Source: CAD feature listing. Evaluate the final solid. Frame: model axes, mm. A direction names the side the tool comes from. Round coordinates to 2 decimals unless told otherwise and drop trailing zeros. Order: outer loops, then holes, each group sorted by start corner. A loop starts at its lowest first (then second) coordinate and runs counter-clockwise, first axis right, second up. Notation, with made-up numbers: (66.5, 58.5) - (101.5, 58.5) arc R18 ccw to (101.5, 88.5) - close; hole circle Ø3 at (-20, -29.75). An arc over 180 degrees is marked (long way). Use one line per item in the form item = value. Start each with the question number.
Q1. Ray query, line 1 (Y direction, x = 0.45, z = 1.5); line 2 (Y direction, x = -0.6, z = -0.55); line 3 (Z direction, x = 0.4, y = 12.75). Return the intervals inside material, ascending. Write a range as [from, to].
Q2. Set-up query: faces 4 (the cylindrical face through (0.45, 7.89, 1.43)), 5 (the flat face through (-0.656, 18.014, -1.349)), 6 (the flat face through (2, 19, 0)). Return all of +Z, -Z, +X, -X, +Y, -Y with unobstructed straight access to the full face (end or side cutting, diameter ignored); none if empty.
Q3. Pin query (flat end, axial travel): pin 1 Ø2 at (y, z) = (10.5, -2) entering from -X. Return the tip coordinate at first contact, or that it passes through.
Q4. Draft query along Z for faces 1 (the cylindrical face through (-2.44, 16.99, -0.54)), 2 (the flat face through (-2, 16, 0)), 3 (the flat face through (0.841, 18.014, -1.242)). Return one class per face: released by +Z, released by -Z, zero draft, split by the parting line, or undercut.
Q5. Cut plane B-B, the plane z = 0. Return the cut outline in (x, y).
Q6. Cut plane A-A, the plane y = 17.25. Return the cut outline in (x, z).
Q7. Cut plane C-C, the plane y = 12.5. Return the cut outline in (x, z), and give its area (3 significant figures).
from build123d import *

# Parameters (mm, degrees)
SKICA1_R                 = 1.5
P_IDAT_VYSUNUT_M1_DEPTH  = 16
SKICA2_R                 = 2.5
P_IDAT_VYSUNUT_M2_DEPTH  = 3
ZKOSEN_1_SIZE            = 1
ZKOSEN_1_SIZE2           = 0.267949192
ODEBRAT_VYSUNUT_M1_DEPTH = 2


with BuildPart() as part:
    # Skica1 → Přidat vysunutím1 (new body)
    with BuildSketch(Plane(origin=(0, 0, 0), x_dir=(1, 0, 0), z_dir=(0, 1, 0))):
        with Locations(Location((0, 0, 0), (0, 0, 270))):
            Circle(SKICA1_R)
    extrude(amount=P_IDAT_VYSUNUT_M1_DEPTH)

    # Skica2 → Přidat vysunutím2 (add)
    with BuildSketch(Plane(origin=(0, 16, 0), x_dir=(1, 0, 0), z_dir=(0, 1, 0))):
        with Locations(Location((0, 0, 0), (0, 0, 270))):
            Circle(SKICA2_R)
    extrude(amount=P_IDAT_VYSUNUT_M2_DEPTH)

    # Zkosení1
    zkosen_1_edges = [part.edges().sort_by_distance(p)[0] for p in [
        (0, 19, -2.5),
    ]]
    zkosen_1_side = [part.faces().sort_by_distance(p)[0] for p in [
        (0, 17.5, -2.5),
    ]]
    chamfer(zkosen_1_edges, length=ZKOSEN_1_SIZE, length2=ZKOSEN_1_SIZE2, reference=zkosen_1_side[0])

    # Skica3 → Odebrat vysunutím1 (cut)
    with BuildSketch(Plane(origin=(0, 19, 0), x_dir=(1, 0, 0), z_dir=(0, 1, 0))):
        Polygon((-0.109437804, -1.728589994), (1.442283945, -0.959070916), (1.55172175, 0.769519078), (0.109437804, 1.728589994), (-1.442283945, 0.959070916), (-1.55172175, -0.769519078), align=None)
    extrude(amount=-ODEBRAT_VYSUNUT_M1_DEPTH, mode=Mode.SUBTRACT)


solid = part.part
Completed:
q1.line_1 = [16, 19]
q1.line_2 = [0, 17]
q1.line_3 = [-1.45, 1.45]
q2.face_4 = -Y
q2.face_5 = +Y
q2.face_6 = +Z, -Z, +X, -X, +Y
q3.pin_1 = -1.12
q4.face_1 = split by the parting line
q4.face_2 = zero draft
q4.face_3 = undercut
q5.outline = (-2.5, 16) - (-1.5, 16) - (-1.5, 0) - (1.5, 0) - (1.5, 16) - (2.5, 16) - (2.5, 18) - (2.23, 19) - (1.5, 19) - (1.5, 17) - (-1.5, 17) - (-1.5, 19) - (-2.23, 19) - (-2.5, 18) - close
q6.outline = circle Ø5 at (0, 0); hole (-1.55, 0.77) - (-1.44, -0.96) - (0.11, -1.73) - (1.55, -0.77) - (1.44, 0.96) - (-0.11, 1.73) - close
q7.outline = circle Ø3 at (0, 0)
q7.area = 7.07 mm2
